For this review, take the finished solid that the model builds, in its own axes (mm). Round coordinates to 2 decimals unless told otherwise and drop trailing zeros. Order: outer loops, then holes, each group sorted by start corner. A loop starts at its lowest first (then second) coordinate and runs counter-clockwise, first axis right, second up. Notation, with made-up numbers: (-26, -6.5) -> (23, -6.5) arc R14 ccw to (23, 11.5) -> close; hole circle Ø8 at (30.25, 62.5). An arc over 180 degrees is marked (long way). Use a Markdown table: item, result. Add a question column.
1) Consider section A-A (x = 0). State the section outline as (y, z) points (3 decimals), plus the area to 3 significant figures.
2) Consider section C-C (z = 16). State the section outline as (x, y) points.
3) Draft analysis for pull direction Z (two halves, no side actions). For faces 1 (the face through (-8, 6.35, 0)), 2 (the face through (-6.883, 3.131, 30.995)), 3 (the face through (8.504, 3.219, 4.874)), state which applies: pulls with the +Z half, pulls with the -Z half, needs draft (parallel to the pull), parting line crosses it, or undercut.
4) Consider section D-D (y = 5). Give the number of separate pieces and of enclosed holes in the cut face, plus the area to 3 significant figures.
5) Consider section B-B (z = -3.5). State the section outline as (x, y) points, plus the area to 3 significant figures.
6) Wall thickness on line 1 along X through (y, z) = (5.5, -12); line 2 along Z through (x, y) = (-8, 2.75); line 3 along X through (y, z) = (1.5, -15): over which ranges is each line inside the solid? List them lowest first. Write a range as [from, to].
7) Clearance check with flat-ended pins moving along their axes: P1, Ø1.9, axis at y = 2.5, z = 16, coming from the +X side; P2, Ø1.4, axis at x = 6.35, z = 0, coming from the +Y side; P3, Ø1.9, axis at y = 4.5, z = 17.5, coming from the -X side; P4, Ø3, axis at x = -0.5, y = 3, coming from the +Z side. State where each tip first meets the part, or that it passes through.
```python
from build123d import *

# Parameters (mm, degrees)
SKETCH1_R           = 31.75
SKETCH1_R_2         = 1.1303
BOSS_EXTRUDE1_DEPTH = 6.35
SKETCH2_R           = 25.4
SKETCH2_R_2         = 9.525
CUT_EXTRUDE1_DEPTH  = 6.35
BOSS_EXTRUDE2_DEPTH = 6.35
CIRPATTERN1_COUNT   = 5


with BuildPart() as part:
    # Sketch1 → Boss-Extrude1 (new body)
    with BuildSketch(Plane(origin=(0, 0, 0), x_dir=(1, 0, 0), z_dir=(0, 1, 0))):
        Circle(SKETCH1_R)
        with Locations((-6.35, 0)):
            Circle(SKETCH1_R_2, mode=Mode.SUBTRACT)
        with Locations((0, 6.35)):
            Circle(SKETCH1_R_2, mode=Mode.SUBTRACT)
        with Locations((6.35, 0)):
            Circle(SKETCH1_R_2, mode=Mode.SUBTRACT)
        with Locations((0, -6.35)):
            Circle(SKETCH1_R_2, mode=Mode.SUBTRACT)
        with BuildLine():
            Line((-1.322875656, 1.5), (1.322875656, 1.5))
            ThreePointArc((1.322875656, 1.5), (0, -2), (-1.322875656, 1.5))
        make_face(mode=Mode.SUBTRACT)
    extrude(amount=BOSS_EXTRUDE1_DEPTH)

    # Sketch2 → Cut-Extrude1 (cut)
    with BuildSketch(Plane(origin=(0, 6.35, 0), x_dir=(1, 0, 0), z_dir=(0, 1, 0))):
        Circle(SKETCH2_R)
        Circle(SKETCH2_R_2, mode=Mode.SUBTRACT)
    extrude(amount=-CUT_EXTRUDE1_DEPTH, mode=Mode.SUBTRACT)

    # Sketch3 → Boss-Extrude2 (add)
    with BuildSketch(Plane(origin=(0, 6.35, 0), x_dir=(1, 0, 0), z_dir=(0, 1, 0))):
        with BuildLine():
            Line((-1.74625, -10.365049973), (-1.74625, -23.940742176))
            ThreePointArc((-1.74625, -23.940742176), (-2.176223959, -24.893242176), (-3.175, -25.200781238))
            ThreePointArc((-3.175, -25.200781238), (0, -25.4), (3.175, -25.200781238))
            ThreePointArc((3.175, -25.200781238), (2.176223959, -24.893242176), (1.74625, -23.940742176))
            Line((1.74625, -23.940742176), (1.74625, -10.365049973))
            ThreePointArc((1.74625, -10.365049973), (2.000483483, -9.602738762), (2.661397059, -9.145632329))
            ThreePointArc((2.661397059, -9.145632329), (0, -9.525), (-2.661397059, -9.145632329))
            ThreePointArc((-2.661397059, -9.145632329), (-2.000483483, -9.602738762), (-1.74625, -10.365049973))
        make_face()
    boss_extrude2 = extrude(amount=-BOSS_EXTRUDE2_DEPTH)

    # CirPattern1: Boss-Extrude2 ×5 about axis
    cirpattern1_axis = Axis((0, 0, 0), (0, 1, 0))
    for i in range(1, CIRPATTERN1_COUNT):
        add(boss_extrude2.rotate(cirpattern1_axis, i * 360 / CIRPATTERN1_COUNT))


solid = part.part
```
Results list:
| question | item | result |
|---|---|---|
| 1 | outline | (0, -31.75) -> (6.35, -31.75) -> (6.35, -25.4) -> (0, -25.4) -> close; (0, -9.525) -> (6.35, -9.525) -> (6.35, -7.48) -> (0, -7.48) -> close; (0, -5.22) -> (6.35, -5.22) -> (6.35, -1.5) -> (0, -1.5) -> close; (0, 2) -> (6.35, 2) -> (6.35, 5.22) -> (0, 5.22) -> close; (0, 7.48) -> (6.35, 7.48) -> (6.35, 31.75) -> (0, 31.75) -> close |
| 1 | area | 251 mm2 |
| 2 | outline | (-27.42, 0) -> (-19.73, 0) -> (-19.73, 6.35) -> (-27.42, 6.35) -> close; (-1.75, 0) -> (1.75, 0) -> (1.75, 6.35) -> (-1.75, 6.35) -> close; (19.73, 0) -> (27.42, 0) -> (27.42, 6.35) -> (19.73, 6.35) -> close |
| 3 | face 1 | needs draft |
| 3 | face 2 | parting line crosses it |
| 3 | face 3 | undercut |
| 4 | separate pieces | 1 |
| 4 | enclosed holes | 10 |
| 4 | area | 1,680 mm2 |
| 5 | outline | (-31.56, 0) -> (-25.16, 0) -> (-25.16, 6.35) -> (-31.56, 6.35) -> close; (-8.86, 0) -> (8.86, 0) -> (8.86, 6.35) -> (-8.86, 6.35) -> close; (25.16, 0) -> (31.56, 0) -> (31.56, 6.35) -> (25.16, 6.35) -> close |
| 5 | area | 194 mm2 |
| 6 | line 1 | [-29.39, -22.39], [-10.88, -6.56], [6.56, 10.88], [22.39, 29.39] |
| 6 | line 2 | [-30.73, -24.11], [-13.98, -8.04], [-5.17, 5.2], [24.11, 30.73] |
| 6 | line 3 | [-27.98, -20.5], [-13.06, -8.74], [8.74, 13.06], [20.5, 27.98] |
| 7 | P1 | x = 27.96 |
| 7 | P2 | through |
| 7 | P3 | x = -27.1 |
| 7 | P4 | z = 31.75 |
